from build123d import *

# Parameters (mm, degrees)
HOLE_WIZARD_M101_D     = 8.5
HOLE_WIZARD_M101_DEPTH = 52.5
HOLE_WIZARD_M101_TIP   = 2.553657631
CHAMFER_1_SIZE         = 1
CUT_EXTRUDE_START      = 22.5
CUT_EXTRUDE_1_DEPTH    = 5.5
CUT_EXTRUDE_2_DEPTH    = 5.5


with BuildPart() as part:
    # Эскиз1 → Повернуть1 (revolve)
    with BuildSketch(Plane.XY, mode=Mode.PRIVATE) as revolve_1_sk:
        Polygon((0, 0), (0, 22.5), (170, 22.5), (170, 25), (180, 25), (180, 22.5), (250, 22.5), (250, 0), align=None)
    revolve(revolve_1_sk.sketch.rotate(Axis((0, 0, 0), (-1, 0, 0)), 90), axis=Axis((0, 0, 0), (-1, 0, 0)))

    # Отверстие обработанное метчиком M101
    with Locations(Plane.ZY):
        with Locations((0, 0)):
            Hole(HOLE_WIZARD_M101_D / 2, depth=HOLE_WIZARD_M101_DEPTH)
            with Locations((0, 0, -(HOLE_WIZARD_M101_DEPTH + HOLE_WIZARD_M101_TIP / 2))):  # 118° drill point
                Cone(0, HOLE_WIZARD_M101_D / 2, HOLE_WIZARD_M101_TIP, mode=Mode.SUBTRACT)

    # Фаска1
    chamfer_1_edges = [part.edges().sort_by_distance(p)[0] for p in [
        (250, 0, 22.5),
        (180, 0, 25),
        (170, 0, 25),
        (0, 0, 22.5),
    ]]
    chamfer(chamfer_1_edges, length=CHAMFER_1_SIZE)

    # Эскиз4 → Вырез-Вытянуть1 (cut)
    with BuildSketch(Plane.XY.offset(CUT_EXTRUDE_START)):
        with BuildLine():
            Line((237.5, -7), (191.5, -7))
            ThreePointArc((191.5, -7), (184.5, 0), (191.5, 7))
            Line((191.5, 7), (237.5, 7))
            ThreePointArc((237.5, 7), (244.5, 0), (237.5, -7))
        make_face()
    extrude(amount=-CUT_EXTRUDE_1_DEPTH, mode=Mode.SUBTRACT)

    # Эскиз5 → Вырез-Вытянуть2 (cut)
    with BuildSketch(Plane.XY.offset(CUT_EXTRUDE_START)):
        with BuildLine():
            Line((17, 7), (153, 7))
            ThreePointArc((153, 7), (160, 0), (153, -7))
            Line((153, -7), (17, -7))
            ThreePointArc((17, -7), (10, 0), (17, 7))
        make_face()
    extrude(amount=-CUT_EXTRUDE_2_DEPTH, mode=Mode.SUBTRACT)


solid = part.part
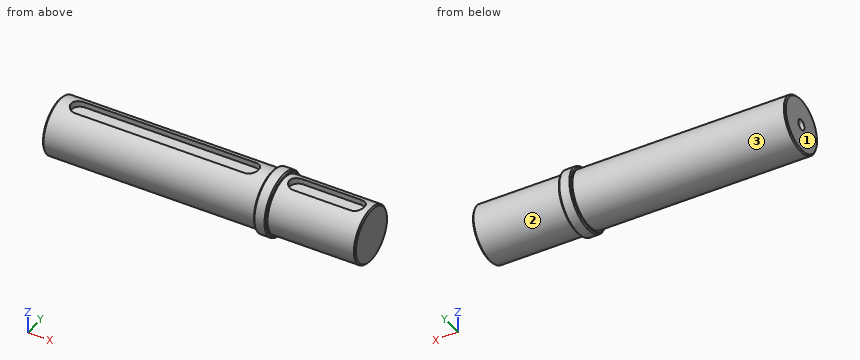
Could you check a few things on this model? Use its own coordinates, in mm. Face numbers are marked on the shaded views. A direction names the side the tool comes from. Give positions to 0.01 mm unless a question says otherwise; leave off trailing zeros. Order: outer loops, then holes, each group sorted by start corner. A loop starts at its lowest first (then second) coordinate and runs counter-clockwise, first axis right, second up. Notation, with made-up numbers: (-26.5, 76.5) - (-14.5, 76.5) arc R23 ccw to (-14.5, 93.5) - close; hole circle Ø4 at (-14, 0.5). An arc over 180 degrees is marked (long way). One line per item, written item: value. Start each with the question number.
1. For P1, Ø2, axis at x = 220.5, z = 18.5, coming from the +Y side; P2, Ø5, axis at y = 0, z = 0, coming from the -X side; P3, Ø4, axis at x = 108, y = -3.5, coming from the +Z side, each with a flat end and sliding along its axis, tell me the tip position at first contact or that it passes through.
2. If I drill on probe 1 along Y at (x, z) = (13, 0); probe 2 along X at (y, z) = (-23, 4.5); probe 3 along Z at (x, y) = (136.5, -0.5), over which ranges is the centre line in solid material (lowest first)?
3. For the marked faces 1, 2 and 3, which set-ups out of +Z, -Z, +X, -X, +Y, -Y let a thin tool reach every point of the face, with its end or its side?
4. Imagine slicing it at A-A on x = 206.5. List the corners of the cut face in (y, z) for me, plus the area to 3 significant figures.
Values:
1. P1: y = 14.14
1. P2: x = 53.55
1. P3: z = 17
2. probe 1: -22.5 to -4.25, 4.25 to 22.5
2. probe 2: 170 to 180
2. probe 3: -22.49 to 17
3. face 1: +Z, -Z, -X, +Y, -Y
3. face 2: +X
3. face 3: -X
4. outline: (-7, 17) - (-7, 21.38) arc R22.5 ccw (long way) to (7, 21.38) - (7, 17) - close
4. area: 1,520 mm²
